Geometry check sheet. Reference: the model listing, model coordinates, mm. Face numbers are marked on the shaded views. A direction names the side the tool comes from. Give positions to 0.01 mm unless a question says otherwise; leave off trailing zeros. Loops run counter-clockwise (first coordinate to the right, second up) from the corner with the lowest first, then second, coordinate; pieces in that order, holes last. Notation, with made-up numbers: (17.5, -17.75) -> (26.5, -17.75) arc R21 ccw to (26.5, 19.25) -> close; hole circle Ø8 at (80.5, 50.5). An arc over 180 degrees is marked (long way). Write item = value, one per line.
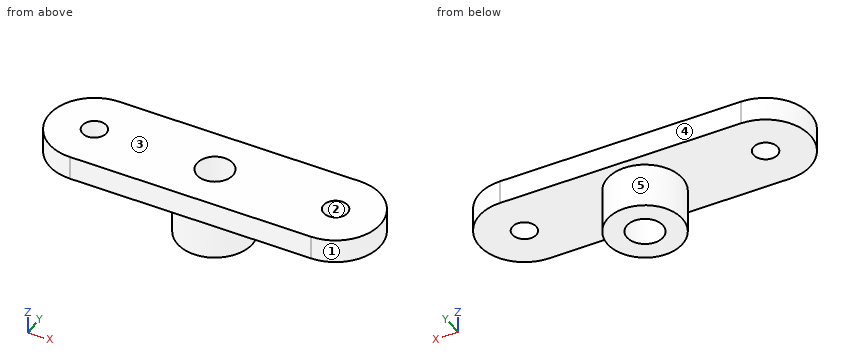
Autodesk Inventor part; units mm, degrees
ref_plane "YZ Plane" through (0, 0, 0) normal (1, 0, 0) x (0, 1, 0)
ref_plane "XZ Plane" through (0, 0, 0) normal (0, 1, 0) x (-1, 0, 0)
ref_plane "XY Plane" through (0, 0, 0) normal (0, 0, 1) x (1, 0, 0)
sketch "Эскиз1" plane through (0, 0, 0) normal (0, 0, 1) x (1, 0, 0)
  line L0 (-40, 0) -> (40, 0) construction
  line L1 (-40, -15) -> (40, -15)
  line L2 (40, 15) -> (-40, 15)
  arc A0 (-40, 15) -> (-40, -15) centre (-40, 0) ccw
  arc A1 (40, -15) -> (40, 15) centre (40, 0) ccw
  circle A2 centre (0, 0) radius 12.5
  circle A3 centre (-40, 0) radius 5
  circle A4 centre (40, 0) radius 5
  circle A5 centre (0, 0) radius 6
  dimension "d1" = 30
  dimension "d2" = 80
  dimension "d5" = 25
  dimension "d6" = 10
  dimension "d7" = 10
  dimension "d8" = 12
extrude "Выдавливание1" add sketch "Эскиз1" along normal blind 8 contours A0 L2 A1 L1 | A2 | A3 | A4 | A5
hole "Отверстие1" at (40, 0, 0) direction (0, 0, 1) diameter 8 end through all
hole "Отверстие2" at (-40, 0, 0) direction (0, 0, 1) diameter 8 end through all
extrude "Выдавливание2" add sketch "Эскиз1" against normal blind 15 contours A2
extrude "Выдавливание3" cut sketch "Эскиз1" along normal blind 15 contours A5
equation "\"Радиус_гибки\" = Толщина"
equation "\"Ширина_просечки\" = Толщина"
equation "\"Глубина_просечки\" = 0.5 * Толщина"
equation "\"Размер_просечки\" = 4 * Толщина"
equation "\"Мин_остаток\" = 2 * Толщина"
equation "\"Радиус_перехода\" = Радиус_гибки"
equation "\"Радиус_Якоби\" = Толщина"
equation "\"Размер_зазора\" = Толщина"
properties part number "pr3defauldetail" material "Нержавеющая сталь"
Item 1: Tool access check on the marked faces 4 and 5. Record the directions out of +Z, -Z, +X, -X, +Y, -Y that give a thin tool (end or side, any length) a straight path to the whole face; none if there is none.
Answer:
face_4 = +Z, -Z, +X, -X, +Y
face_5 = -Z
Item 2: Section check D-D, the plane y = -7.25. Record the cut outline in (x, z), plus the area to 3 significant figures.
Answer:
outline = (-53.13, 0) -> (-10.18, 0) -> (-10.18, -15) -> (10.18, -15) -> (10.18, 0) -> (53.13, 0) -> (53.13, 8) -> (-53.13, 8) -> close
area = 1,160 mm^2
Item 3: Gauge pin test, flat ends, axial feed: pin 1 (2 mm diameter, centred on x = 35.5, z = -2, fed in from +Y); pin 2 (6 mm diameter, centred on x = 0.5, z = -9, fed in from +Y); pin 3 (1.5 mm diameter, centred on x = 16, y = 0, fed in from -Z). Record the tip position at first contact, or that the pin passes through.
Answer:
pin_1 = through
pin_2 = 12.5
pin_3 = 0
Item 4: Section check A-A, the plane y = 0. Record the cut outline in (x, z), plus the area to 3 significant figures.
Answer:
outline = (-55, 0) -> (-44, 0) -> (-44, 8) -> (-55, 8) -> close; (-36, 0) -> (-12.5, 0) -> (-12.5, -15) -> (-6, -15) -> (-6, 8) -> (-36, 8) -> close; (6, -15) -> (12.5, -15) -> (12.5, 0) -> (36, 0) -> (36, 8) -> (6, 8) -> close; (44, 0) -> (55, 0) -> (55, 8) -> (44, 8) -> close
area = 851 mm^2
Item 5: Section check C-C, the plane z = -3. Record the cut outline in (x, y), plus the area to 3 significant figures.
Answer:
outline = circle Ø25 at (0, 0); hole circle Ø12 at (0, 0)
area = 378 mm^2
Item 6: Draft check along X on the marked faces 1, 2 and 3. Enter one of: +X half, -X half, draft (parallel to the pull), parting line (faces both ways), or undercut.
Answer:
face_1 = +X half
face_2 = undercut
face_3 = draft
Item 7: Thickness scan on L1, parallel to X at y = 0, z = 3; L2, parallel to Y at x = -40, z = 4.5; L3, parallel to Y at x = -1, z = -14. Record the ranges inside material, lowest first. Write a range as [from, to].
Answer:
L1 = [-55, -44], [-36, -6], [6, 36], [44, 55]
L2 = [-15, -4], [4, 15]
L3 = [-12.46, -5.92], [5.92, 12.46]
Item 8: Section check B-B, the plane x = 0. Record the cut outline in (y, z), plus the area to 3 significant figures.
Answer:
outline = (-15, 0) -> (-12.5, 0) -> (-12.5, -15) -> (-6, -15) -> (-6, 8) -> (-15, 8) -> close; (6, -15) -> (12.5, -15) -> (12.5, 0) -> (15, 0) -> (15, 8) -> (6, 8) -> close
area = 339 mm^2
